from build123d import *

# Parameters (mm, degrees)
SKETCH1_R          = 2.15
SKETCH1_R_2        = 2
EXTRUDE1_DEPTH     = 2
FILLET1_R          = 10
FILLET2_R          = 10
CHAMFER1_SIZE      = 30
SKETCH3_R          = 2.15
CUT_EXTRUDE1_DEPTH = 3
CUT_EXTRUDE2_DEPTH = 10


with BuildPart() as part:
    # Sketch1 → Extrude1 (new body)
    # profile 1 of 2: a face of its own
    with BuildSketch(Plane.XY):
        with BuildLine():
            Line((-17.67766953, 17.67766953), (-56.568542495, 56.568542495))
            Line((-56.568542495, 56.568542495), (-107.833729857, 5.303355133))
            Line((-107.833729857, 5.303355133), (-121.975865481, 19.445490757))
            Line((-121.975865481, 19.445490757), (-157.33120454, -15.909848303))
            Line((-157.33120454, -15.909848303), (-129.046933293, -44.19411955))
            Line((-129.046933293, -44.19411955), (-102.530428998, -17.677615256))
            Line((-102.530428998, -17.677615256), (-84.852759469, -35.355284785))
            Line((-84.852759469, -35.355284785), (-111.369263763, -61.87178908))
            Line((-111.369263763, -61.87178908), (-110.869178063, -62.37187478))
            Line((-110.869178063, -62.37187478), (-61.87178908, -111.369263763))
            Line((-61.87178908, -111.369263763), (-35.355284785, -84.852759468))
            Line((-35.355284785, -84.852759468), (-17.677615256, -102.530428998))
            Line((-17.677615256, -102.530428998), (-44.19411955, -129.046933293))
            Line((-44.19411955, -129.046933293), (-30.051983927, -143.189068916))
            Line((-30.051983927, -143.189068916), (56.568542495, -56.568542495))
            Line((56.568542495, -56.568542495), (17.67766953, -17.67766953))
            ThreePointArc((17.67766953, -17.67766953), (-17.67766953, -17.67766953), (-17.67766953, 17.67766953))
        make_face()
        with Locations((-54.5, 0)):
            Circle(SKETCH1_R, mode=Mode.SUBTRACT)
        with Locations((0, -54.5)):
            Circle(SKETCH1_R, mode=Mode.SUBTRACT)
        with Locations((21.294846503, -50.167514513)):
            Circle(SKETCH1_R_2, mode=Mode.SUBTRACT)
    # profile 2 of 2: a face of its own
    with BuildSketch(Plane.XY):
        with BuildLine():
            Line((17.677615256, 102.530428998), (44.19411955, 129.046933293))
            Line((44.19411955, 129.046933293), (15.909848303, 157.33120454))
            Line((15.909848303, 157.33120454), (-19.445490757, 121.975865481))
            Line((-19.445490757, 121.975865481), (-5.303355133, 107.833729857))
            Line((-5.303355133, 107.833729857), (-56.568542495, 56.568542495))
            Line((-56.568542495, 56.568542495), (-17.67766953, 17.67766953))
            ThreePointArc((-17.67766953, 17.67766953), (9.567085809, 23.096988313), (25, 0))
            ThreePointArc((25, 0), (23.096988313, -9.567085809), (17.67766953, -17.67766953))
            Line((17.67766953, -17.67766953), (56.568542495, -56.568542495))
            Line((56.568542495, -56.568542495), (143.189068916, 30.051983927))
            Line((143.189068916, 30.051983927), (129.046933293, 44.19411955))
            Line((129.046933293, 44.19411955), (102.530428998, 17.677615256))
            Line((102.530428998, 17.677615256), (84.852759469, 35.355284785))
            Line((84.852759469, 35.355284785), (111.369263763, 61.87178908))
            Line((111.369263763, 61.87178908), (61.87178908, 111.369263763))
            Line((61.87178908, 111.369263763), (35.355284785, 84.852759469))
            Line((35.355284785, 84.852759469), (17.677615256, 102.530428998))
        make_face()
        with Locations((50.167514513, -21.294846503)):
            Circle(SKETCH1_R, mode=Mode.SUBTRACT)
        with Locations((54.5, 0)):
            Circle(SKETCH1_R, mode=Mode.SUBTRACT)
        with Locations((0, 54.5)):
            Circle(SKETCH1_R, mode=Mode.SUBTRACT)
    extrude(amount=EXTRUDE1_DEPTH)

    # Fillet1
    fillet1_edges = [part.edges().sort_by_distance(p)[0] for p in [
        (-107.833729857, 5.303355133, 1),
        (-5.303355133, 107.833729857, 1),
    ]]
    fillet(fillet1_edges, radius=FILLET1_R)

    # Fillet2
    fillet2_edges = [part.edges().sort_by_distance(p)[0] for p in [
        (-17.677615256, -102.530428998, 1),
        (-35.355284785, -84.852759468, 1),
        (-84.852759469, -35.355284785, 1),
        (-102.530428998, -17.677615256, 1),
        (17.677615256, 102.530428998, 1),
        (35.355284785, 84.852759469, 1),
        (84.852759469, 35.355284785, 1),
        (102.530428998, 17.677615256, 1),
    ]]
    fillet(fillet2_edges, radius=FILLET2_R)

    # Chamfer1
    chamfer1_edges = [part.edges().sort_by_distance(p)[0] for p in [
        (-157.33120454, -15.909848303, 1),
        (15.909848303, 157.33120454, 1),
    ]]
    chamfer(chamfer1_edges, length=CHAMFER1_SIZE)

    # Sketch3 → Cut-Extrude1 (cut)
    with BuildSketch(Plane.XY.offset(2)):
        with Locations((130.064043572, 36.323458724)):
            Circle(SKETCH3_R)
        with Locations((36.394169402, 130.13475425)):
            Circle(SKETCH3_R)
        with Locations((-36.3941694, -130.134754248)):
            Circle(SKETCH3_R)
        with Locations((-130.13475425, -36.394169402)):
            Circle(SKETCH3_R)
    extrude(amount=-CUT_EXTRUDE1_DEPTH, mode=Mode.SUBTRACT)

    # Sketch4 → Cut-Extrude2 (cut)
    with BuildSketch(Plane.XY.offset(2)):
        with BuildLine():
            Line((64.700216205, 97.227128139), (97.227128139, 64.700216205))
            ThreePointArc((97.227128139, 64.700216205), (97.227128139, 59.043361955), (91.57027389, 59.043361955))
            Line((91.57027389, 59.043361955), (59.043361955, 91.57027389))
            ThreePointArc((59.043361955, 91.57027389), (59.043361955, 97.227128139), (64.700216205, 97.227128139))
        make_face()
        with BuildLine():
            Line((54.093614487, 86.620526421), (86.620526421, 54.093614487))
            ThreePointArc((86.620526421, 54.093614487), (86.620526421, 48.436760237), (80.963672172, 48.436760237))
            Line((80.963672172, 48.436760237), (48.436760237, 80.963672172))
            ThreePointArc((48.436760237, 80.963672172), (48.436760237, 86.620526421), (54.093614487, 86.620526421))
        make_face()
        with BuildLine():
            Line((43.487012769, 76.013924704), (76.013924704, 43.487012769))
            ThreePointArc((76.013924704, 43.487012769), (76.013924704, 37.83015852), (70.357070454, 37.83015852))
            Line((70.357070454, 37.83015852), (37.83015852, 70.357070454))
            ThreePointArc((37.83015852, 70.357070454), (37.83015852, 76.013924704), (43.487012769, 76.013924704))
        make_face()
        with BuildLine():
            Line((32.880411051, 65.407322986), (65.407322986, 32.880411051))
            ThreePointArc((65.407322986, 32.880411051), (65.407322986, 27.223556802), (59.750468736, 27.223556802))
            Line((59.750468736, 27.223556802), (27.223556802, 59.750468736))
            ThreePointArc((27.223556802, 59.750468736), (27.223556802, 65.407322986), (32.880411051, 65.407322986))
        make_face()
        with BuildLine():
            Line((22.273809333, 54.800721268), (54.800721268, 22.273809333))
            ThreePointArc((54.800721268, 22.273809333), (54.800721268, 16.616955084), (49.143867019, 16.616955084))
            Line((49.143867019, 16.616955084), (16.616955084, 49.143867019))
            ThreePointArc((16.616955084, 49.143867019), (16.616955084, 54.800721268), (22.273809333, 54.800721268))
        make_face()
        with BuildLine():
            Line((-97.227128139, -64.700216205), (-64.700216205, -97.227128139))
            ThreePointArc((-64.700216205, -97.227128139), (-59.043361955, -97.227128139), (-59.043361955, -91.57027389))
            Line((-59.043361955, -91.57027389), (-91.57027389, -59.043361955))
            ThreePointArc((-91.57027389, -59.043361955), (-97.227128139, -59.043361955), (-97.227128139, -64.700216205))
        make_face()
        with BuildLine():
            Line((-86.620526421, -54.093614487), (-54.093614487, -86.620526421))
            ThreePointArc((-54.093614487, -86.620526421), (-48.436760237, -86.620526421), (-48.436760237, -80.963672172))
            Line((-48.436760237, -80.963672172), (-80.963672172, -48.436760237))
            ThreePointArc((-80.963672172, -48.436760237), (-86.620526421, -48.436760237), (-86.620526421, -54.093614487))
        make_face()
        with BuildLine():
            Line((-76.013924704, -43.487012769), (-43.487012769, -76.013924704))
            ThreePointArc((-43.487012769, -76.013924704), (-37.83015852, -76.013924704), (-37.83015852, -70.357070454))
            Line((-37.83015852, -70.357070454), (-70.357070454, -37.83015852))
            ThreePointArc((-70.357070454, -37.83015852), (-76.013924704, -37.83015852), (-76.013924704, -43.487012769))
        make_face()
        with BuildLine():
            Line((-65.407322986, -32.880411051), (-32.880411051, -65.407322986))
            ThreePointArc((-32.880411051, -65.407322986), (-27.223556802, -65.407322986), (-27.223556802, -59.750468736))
            Line((-27.223556802, -59.750468736), (-59.750468736, -27.223556802))
            ThreePointArc((-59.750468736, -27.223556802), (-65.407322986, -27.223556802), (-65.407322986, -32.880411051))
        make_face()
        with BuildLine():
            Line((-54.800721268, -22.273809333), (-22.273809333, -54.800721268))
            ThreePointArc((-22.273809333, -54.800721268), (-16.616955084, -54.800721268), (-16.616955084, -49.143867019))
            Line((-16.616955084, -49.143867019), (-49.143867019, -16.616955084))
            ThreePointArc((-49.143867019, -16.616955084), (-54.800721268, -16.616955084), (-54.800721268, -22.273809333))
        make_face()
    extrude(amount=-CUT_EXTRUDE2_DEPTH, mode=Mode.SUBTRACT)


solid = part.part
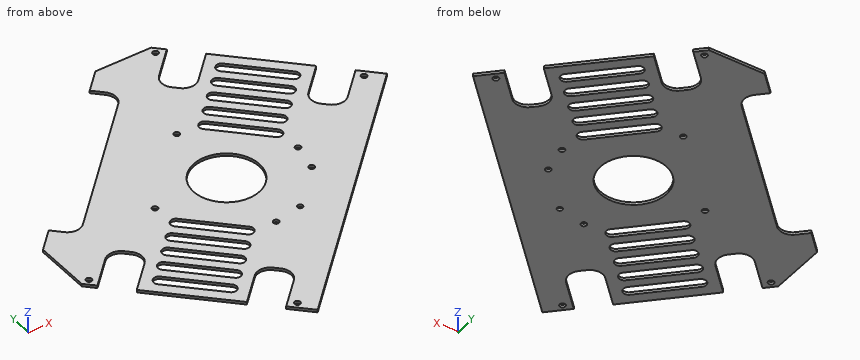
Can you work these out from the model? Positions are in its coordinate system, mm. Give positions to 0.01 mm unless a question says otherwise; leave off trailing zeros. Write each loop counter-clockwise with the first axis right and the second up, starting at its lowest first coordinate (ties: lowest second). Pieces come first, ordered by that corner, then holes. Notation, with made-up numbers: M -37,-20.75 L 9,-20.75 A13 cw 9,-1.75 Z; hole C 84,11 d2. An arc over 180 degrees is marked long. Answer in a Markdown table with one row per item. Add a question column.
Item 1: Please list where these lines run through material, in increasing order: L1, parallel to X at y = 97, z = 1.3; L2, parallel to Y at x = 0, z = 0.8; L3, parallel to Y at x = 67.5, z = 1.2.
Item 2: Imagine slicing it at B-B, the plane z = 0.7. State how many separate pieces and enclosed holes the cut face has, plus the area to 3 significant figures.
Item 3: Imagine slicing it at A-A, the plane y = -123.5. Write out the boundary of the cut face in (x, z).
Item 4: For pin 1 Ø1 at (y, z) = (-41.5, 1) entering from -X, with a flat end and sliding along its axis, tell me the tip position at first contact or that it passes through.
Evaluation:
| question | item | result |
|---|---|---|
| 1 | L1 | x = -16.14 to 23.49, 47.5 to 58.83, 64.93 to 76.24 |
| 1 | L2 | y = -113.14 to -56.65, -52.35 to -25, 25 to 52.35, 56.65 to 136.12 |
| 1 | L3 | y = -45.64 to 40.69, 52 to 61.9, 73.21 to 83.11, 94.43 to 105.74 |
| 2 | separate pieces | 1 |
| 2 | enclosed holes | 21 |
| 2 | area | 30,500 mm² |
| 3 | outline | M -38.65,0 L -10.36,0 L -10.36,2 L -38.65,2 Z |
| 4 | pin 1 | stops at x = -132.24 |
